The model under review builds one solid part; all positions refer to its coordinate system, in mm. Face numbers are marked on the shaded views. A direction names the side the tool comes from. Give positions to 0.01 mm unless a question says otherwise; leave off trailing zeros. Loops run counter-clockwise (first coordinate to the right, second up) from the corner with the lowest first, then second, coordinate; pieces in that order, holes last. Notation, with made-up numbers: (17.5, -22) -> (30.5, -22) arc R32 cw to (30.5, 12) -> close; hole circle Ø10 at (67.5, 61.25). An arc over 180 degrees is marked (long way). Write each question's results on one line, items separated by ' | '. Start each with the question number.
Q1. Machinability: for the marked faces 1 and 2, which of the approach directions +Z, -Z, +X, -X, +Y, -Y give a long, thin tool a straight path to every point of the face, cutting with its end or side? Answer none if there is none.
Q2. We need section B-B (y = 0). Write out the cut boundary in (x, z).
Q3. We need section A-A (z = 0). Write out the cut boundary in (x, y), plus the area to 3 significant figures.
Q4. Insertion check: pin 1 Ø1.5 at (y, z) = (0.5, 0) entering from -X; pin 2 Ø1 at (x, z) = (3.5, 0) entering from +Y. Each pin has a flat end and moves straight along its axis. Give the tip position at first contact, or say it passes through.
Q5. Wall thickness on L1, parallel to X at y = 0.7, z = 0.85; L2, parallel to X at y = -0.05, z = -1.35; L3, parallel to Y at x = 0.5, z = -1.1: over which ranges is each line inside the solid? List them lowest first. Write a range as [from, to].
Q6. We need section C-C (x = 8). Write out the cut boundary in (y, z), plus the area to 3 significant figures.
from build123d import *

# Parameters (mm, degrees)
FILLET1_R     = 0.1
HEAD_RADIUS_R = 0.5
SLOTSKE_W     = 3.2
SLOTSKE_H     = 0.4
SLOT_DEPTH    = 0.35


with BuildPart() as part:
    # BodySke → BaseBody (revolve)
    with BuildSketch(Plane.XY, mode=Mode.PRIVATE) as basebody_sk:
        Polygon((0, 0), (0, 1.512511336), (1, 1.6), (1, 0.8), (11, 0.8), (11, 0), align=None)
    revolve(basebody_sk.sketch.rotate(Axis((0, 0, 0), (1, 0, 0)), 90), axis=Axis((0, 0, 0), (1, 0, 0)))

    # Fillet1
    fillet1_edges = [part.edges().sort_by_distance(p)[0] for p in [
        (1, 0, -0.8),
    ]]
    fillet(fillet1_edges, radius=FILLET1_R)

    # Head_Radius
    head_radius_edges = [part.edges().sort_by_distance(p)[0] for p in [
        (0, 0, -1.512511336),
    ]]
    fillet(head_radius_edges, radius=HEAD_RADIUS_R)

    # SlotSke → Slot (cut)
    with BuildSketch(Plane(origin=(0, 0, 0), x_dir=(0, 0, -1), z_dir=(1, 0, 0))):
        Rectangle(SLOTSKE_W, SLOTSKE_H)
    extrude(amount=SLOT_DEPTH, mode=Mode.SUBTRACT)


solid = part.part
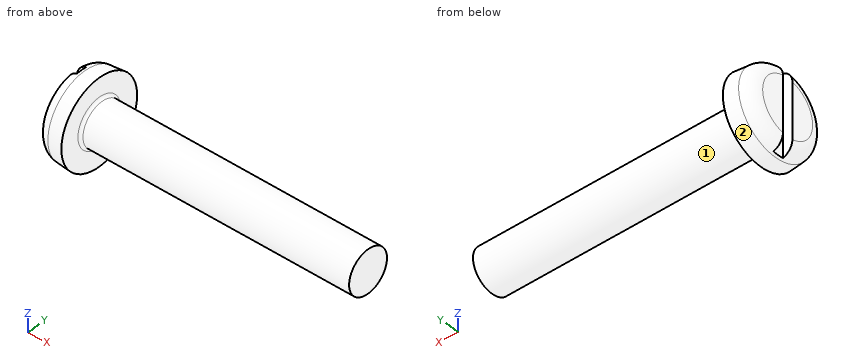
Output:
1) face 1: +X | face 2: -X
2) outline: (0.35, -1.53) arc R0.5 ccw to (0.46, -1.55) -> (1, -1.6) -> (1, -0.9) arc R0.1 cw to (1.1, -0.8) -> (11, -0.8) -> (11, 0.8) -> (1.1, 0.8) arc R0.1 cw to (1, 0.9) -> (1, 1.6) -> (0.46, 1.55) arc R0.5 ccw to (0.35, 1.53) -> close
3) outline: (0, -1.05) arc R0.5 ccw to (0.46, -1.55) -> (1, -1.6) -> (1, -0.9) arc R0.1 cw to (1.1, -0.8) -> (11, -0.8) -> (11, 0.8) -> (1.1, 0.8) arc R0.1 cw to (1, 0.9) -> (1, 1.6) -> (0.46, 1.55) arc R0.5 ccw to (0, 1.05) -> (0, 0.2) -> (0.35, 0.2) -> (0.35, -0.2) -> (0, -0.2) -> close | area: 18.9 mm2
4) pin 1: x = 0 | pin 2: y = 0.8
5) L1: [0, 1] | L2: [0.35, 1] | L3: [-1.1, 1.1]
6) outline: circle Ø1.6 at (0, 0) | area: 2.01 mm2
